```python
from build123d import *

# Parameters (mm, degrees)
SKETCH_1_R             = 2
EXTRUDE_1_DEPTH        = 5
SKETCH_2_R             = 1
CUT_EXTRUDE_1_DEPTH    = 20
PATTERN_LINEAR_1_COUNT = 14
PATTERN_LINEAR_1_PITCH = 15
FILLET_1_R             = 10
SKETCH_3_W             = 6
SKETCH_3_H             = 35
CUT_EXTRUDE_2_DEPTH    = 13
FILLET_2_R             = 3


with BuildPart() as part:
    # 草图1 → 凸台-拉伸1 (new body)
    # profile 1 of 4: a face of its own
    with BuildSketch(Plane.XY):
        with BuildLine():
            ThreePointArc((-33.2, -29.85450543), (-33.123455397, -33.472929676), (-33.700274419, -37.045902236))
            Line((-33.700274419, -37.045902236), (-46.624977248, -87.523440915))
            ThreePointArc((-46.624977248, -87.523440915), (-44.479417414, -97.858032719), (-35, -102.5))
            Line((-35, -102.5), (-5, -102.5))
            Line((-5, -102.5), (5, -102.5))
            Line((5, -102.5), (35, -102.5))
            ThreePointArc((35, -102.5), (44.479417414, -97.858032719), (46.624977248, -87.523440915))
            Line((46.624977248, -87.523440915), (33.700274419, -37.045902236))
            ThreePointArc((33.700274419, -37.045902236), (33.123455397, -33.472929676), (33.2, -29.85450543))
            Line((33.2, -29.85450543), (33.2, 7.364864087))
            Line((33.2, 7.364864087), (5, 41.001264624))
            Line((5, 41.001264624), (5, 99.5))
            ThreePointArc((5, 99.5), (4.121320344, 101.621320344), (2, 102.5))
            Line((2, 102.5), (-2.597497695, 102.5))
            ThreePointArc((-2.597497695, 102.5), (-3.665324968, 102.30352366), (-4.593283712, 101.739829943))
            Line((-4.593283712, 101.739829943), (-33.2, 76.25))
            Line((-33.2, 76.25), (-33.2, -29.85450543))
        make_face()
        with Locations((-42.25, -85.8)):
            Circle(SKETCH_1_R, mode=Mode.SUBTRACT)
        with Locations((-23.75, -85.8)):
            Circle(SKETCH_1_R, mode=Mode.SUBTRACT)
        with Locations((-9.25, -85.8)):
            Circle(SKETCH_1_R, mode=Mode.SUBTRACT)
        with Locations((-26.7, -16.25)):
            Circle(SKETCH_1_R, mode=Mode.SUBTRACT)
        with Locations((9.25, -85.8)):
            Circle(SKETCH_1_R, mode=Mode.SUBTRACT)
        with Locations((23.75, -85.8)):
            Circle(SKETCH_1_R, mode=Mode.SUBTRACT)
        with Locations((42.25, -85.8)):
            Circle(SKETCH_1_R, mode=Mode.SUBTRACT)
        with Locations((26.7, -16.25)):
            Circle(SKETCH_1_R, mode=Mode.SUBTRACT)
        with Locations((-26.7, 2.25)):
            Circle(SKETCH_1_R, mode=Mode.SUBTRACT)
        with Locations((-26.7, 53.751606034)):
            Circle(SKETCH_1_R, mode=Mode.SUBTRACT)
        with Locations((-26.45623641, 72.25)):
            Circle(SKETCH_1_R, mode=Mode.SUBTRACT)
        with Locations((26.7, 2.25)):
            Circle(SKETCH_1_R, mode=Mode.SUBTRACT)
    # profile 2 of 4: a face of its own
    with BuildSketch(Plane.XY):
        with BuildLine():
            ThreePointArc((-33.2, -29.85450543), (-33.123455397, -33.472929676), (-33.700274419, -37.045902236))
            Line((-33.700274419, -37.045902236), (-46.624977248, -87.523440915))
            ThreePointArc((-46.624977248, -87.523440915), (-44.479417414, -97.858032719), (-35, -102.5))
            Line((-35, -102.5), (-5, -102.5))
            Line((-5, -102.5), (5, -102.5))
            Line((5, -102.5), (35, -102.5))
            ThreePointArc((35, -102.5), (44.479417414, -97.858032719), (46.624977248, -87.523440915))
            Line((46.624977248, -87.523440915), (33.700274419, -37.045902236))
            ThreePointArc((33.700274419, -37.045902236), (33.123455397, -33.472929676), (33.2, -29.85450543))
            Line((33.2, -29.85450543), (33.2, 7.364864087))
            Line((33.2, 7.364864087), (5, 41.001264624))
            Line((5, 41.001264624), (5, 99.5))
            ThreePointArc((5, 99.5), (4.121320344, 101.621320344), (2, 102.5))
            Line((2, 102.5), (-2.597497695, 102.5))
            ThreePointArc((-2.597497695, 102.5), (-3.665324968, 102.30352366), (-4.593283712, 101.739829943))
            Line((-4.593283712, 101.739829943), (-33.2, 76.25))
            Line((-33.2, 76.25), (-33.2, -29.85450543))
        make_face()
        with Locations((-42.25, -85.8)):
            Circle(SKETCH_1_R, mode=Mode.SUBTRACT)
        with Locations((-23.75, -85.8)):
            Circle(SKETCH_1_R, mode=Mode.SUBTRACT)
        with Locations((-9.25, -85.8)):
            Circle(SKETCH_1_R, mode=Mode.SUBTRACT)
        with Locations((-26.7, -16.25)):
            Circle(SKETCH_1_R, mode=Mode.SUBTRACT)
        with Locations((9.25, -85.8)):
            Circle(SKETCH_1_R, mode=Mode.SUBTRACT)
        with Locations((23.75, -85.8)):
            Circle(SKETCH_1_R, mode=Mode.SUBTRACT)
        with Locations((42.25, -85.8)):
            Circle(SKETCH_1_R, mode=Mode.SUBTRACT)
        with Locations((26.7, -16.25)):
            Circle(SKETCH_1_R, mode=Mode.SUBTRACT)
        with Locations((-26.7, 2.25)):
            Circle(SKETCH_1_R, mode=Mode.SUBTRACT)
        with Locations((-26.7, 53.751606034)):
            Circle(SKETCH_1_R, mode=Mode.SUBTRACT)
        with Locations((-26.45623641, 72.25)):
            Circle(SKETCH_1_R, mode=Mode.SUBTRACT)
        with Locations((26.7, 2.25)):
            Circle(SKETCH_1_R, mode=Mode.SUBTRACT)
    # profile 3 of 4: a face of its own
    with BuildSketch(Plane.XY):
        with BuildLine():
            ThreePointArc((-33.2, -29.85450543), (-33.123455397, -33.472929676), (-33.700274419, -37.045902236))
            Line((-33.700274419, -37.045902236), (-46.624977248, -87.523440915))
            ThreePointArc((-46.624977248, -87.523440915), (-44.479417414, -97.858032719), (-35, -102.5))
            Line((-35, -102.5), (-5, -102.5))
            Line((-5, -102.5), (5, -102.5))
            Line((5, -102.5), (35, -102.5))
            ThreePointArc((35, -102.5), (44.479417414, -97.858032719), (46.624977248, -87.523440915))
            Line((46.624977248, -87.523440915), (33.700274419, -37.045902236))
            ThreePointArc((33.700274419, -37.045902236), (33.123455397, -33.472929676), (33.2, -29.85450543))
            Line((33.2, -29.85450543), (33.2, 7.364864087))
            Line((33.2, 7.364864087), (5, 41.001264624))
            Line((5, 41.001264624), (5, 99.5))
            ThreePointArc((5, 99.5), (4.121320344, 101.621320344), (2, 102.5))
            Line((2, 102.5), (-2.597497695, 102.5))
            ThreePointArc((-2.597497695, 102.5), (-3.665324968, 102.30352366), (-4.593283712, 101.739829943))
            Line((-4.593283712, 101.739829943), (-33.2, 76.25))
            Line((-33.2, 76.25), (-33.2, -29.85450543))
        make_face()
        with Locations((-42.25, -85.8)):
            Circle(SKETCH_1_R, mode=Mode.SUBTRACT)
        with Locations((-23.75, -85.8)):
            Circle(SKETCH_1_R, mode=Mode.SUBTRACT)
        with Locations((-9.25, -85.8)):
            Circle(SKETCH_1_R, mode=Mode.SUBTRACT)
        with Locations((-26.7, -16.25)):
            Circle(SKETCH_1_R, mode=Mode.SUBTRACT)
        with Locations((9.25, -85.8)):
            Circle(SKETCH_1_R, mode=Mode.SUBTRACT)
        with Locations((23.75, -85.8)):
            Circle(SKETCH_1_R, mode=Mode.SUBTRACT)
        with Locations((42.25, -85.8)):
            Circle(SKETCH_1_R, mode=Mode.SUBTRACT)
        with Locations((26.7, -16.25)):
            Circle(SKETCH_1_R, mode=Mode.SUBTRACT)
        with Locations((-26.7, 2.25)):
            Circle(SKETCH_1_R, mode=Mode.SUBTRACT)
        with Locations((-26.7, 53.751606034)):
            Circle(SKETCH_1_R, mode=Mode.SUBTRACT)
        with Locations((-26.45623641, 72.25)):
            Circle(SKETCH_1_R, mode=Mode.SUBTRACT)
        with Locations((26.7, 2.25)):
            Circle(SKETCH_1_R, mode=Mode.SUBTRACT)
    # profile 4 of 4: a face of its own
    with BuildSketch(Plane.XY):
        with BuildLine():
            ThreePointArc((-33.2, -29.85450543), (-33.123455397, -33.472929676), (-33.700274419, -37.045902236))
            Line((-33.700274419, -37.045902236), (-46.624977248, -87.523440915))
            ThreePointArc((-46.624977248, -87.523440915), (-44.479417414, -97.858032719), (-35, -102.5))
            Line((-35, -102.5), (-5, -102.5))
            Line((-5, -102.5), (5, -102.5))
            Line((5, -102.5), (35, -102.5))
            ThreePointArc((35, -102.5), (44.479417414, -97.858032719), (46.624977248, -87.523440915))
            Line((46.624977248, -87.523440915), (33.700274419, -37.045902236))
            ThreePointArc((33.700274419, -37.045902236), (33.123455397, -33.472929676), (33.2, -29.85450543))
            Line((33.2, -29.85450543), (33.2, 7.364864087))
            Line((33.2, 7.364864087), (5, 41.001264624))
            Line((5, 41.001264624), (5, 99.5))
            ThreePointArc((5, 99.5), (4.121320344, 101.621320344), (2, 102.5))
            Line((2, 102.5), (-2.597497695, 102.5))
            ThreePointArc((-2.597497695, 102.5), (-3.665324968, 102.30352366), (-4.593283712, 101.739829943))
            Line((-4.593283712, 101.739829943), (-33.2, 76.25))
            Line((-33.2, 76.25), (-33.2, -29.85450543))
        make_face()
        with Locations((-42.25, -85.8)):
            Circle(SKETCH_1_R, mode=Mode.SUBTRACT)
        with Locations((-23.75, -85.8)):
            Circle(SKETCH_1_R, mode=Mode.SUBTRACT)
        with Locations((-9.25, -85.8)):
            Circle(SKETCH_1_R, mode=Mode.SUBTRACT)
        with Locations((-26.7, -16.25)):
            Circle(SKETCH_1_R, mode=Mode.SUBTRACT)
        with Locations((9.25, -85.8)):
            Circle(SKETCH_1_R, mode=Mode.SUBTRACT)
        with Locations((23.75, -85.8)):
            Circle(SKETCH_1_R, mode=Mode.SUBTRACT)
        with Locations((42.25, -85.8)):
            Circle(SKETCH_1_R, mode=Mode.SUBTRACT)
        with Locations((26.7, -16.25)):
            Circle(SKETCH_1_R, mode=Mode.SUBTRACT)
        with Locations((-26.7, 2.25)):
            Circle(SKETCH_1_R, mode=Mode.SUBTRACT)
        with Locations((-26.7, 53.751606034)):
            Circle(SKETCH_1_R, mode=Mode.SUBTRACT)
        with Locations((-26.45623641, 72.25)):
            Circle(SKETCH_1_R, mode=Mode.SUBTRACT)
        with Locations((26.7, 2.25)):
            Circle(SKETCH_1_R, mode=Mode.SUBTRACT)
    extrude(amount=EXTRUDE_1_DEPTH)

    # 草图2 → 切除-拉伸1 (cut)
    with BuildSketch(Plane.XY):
        with Locations((0, 97.5)):
            Circle(SKETCH_2_R)
    cut_extrude_1 = extrude(amount=CUT_EXTRUDE_1_DEPTH, mode=Mode.SUBTRACT)

    # 阵列(线性)1: 切除-拉伸1 ×14
    with Locations(*[(0, -i * PATTERN_LINEAR_1_PITCH, 0) for i in range(1, PATTERN_LINEAR_1_COUNT)]):
        add(cut_extrude_1, mode=Mode.SUBTRACT)

    # 圆角1
    fillet_1_edges = [part.edges().sort_by_distance(p)[0] for p in [
        (-33.2, 76.25, 2.5),
        (5, 41.001264624, 2.5),
        (33.2, 7.364864087, 2.5),
    ]]
    fillet(fillet_1_edges, radius=FILLET_1_R)

    # 草图3 → 切除-拉伸2 (cut)
    with BuildSketch(Plane.XY):
        with Locations((-30.2, 28.069279085)):
            Rectangle(SKETCH_3_W, SKETCH_3_H)
    extrude(amount=CUT_EXTRUDE_2_DEPTH, mode=Mode.SUBTRACT)

    # 圆角2
    fillet_2_edges = [part.edges().sort_by_distance(p)[0] for p in [
        (-27.2, 45.569279085, 2.5),
        (-27.2, 10.569279085, 2.5),
    ]]
    fillet(fillet_2_edges, radius=FILLET_2_R)
    fillet_2_2_edges = [part.edges().sort_by_distance(p)[0] for p in [
        (-33.2, 45.569279085, 2.5),
        (-33.2, 10.569279085, 2.5),
    ]]
    fillet(fillet_2_2_edges, radius=FILLET_2_R - 0.0001)  # a hair under: the kernel refuses the full size


solid = part.part
```
Work out the finished part from the listing and answer in its coordinate system (mm). A direction names the side the tool comes from. Round coordinates to 2 decimals unless told otherwise and drop trailing zeros. Loops run counter-clockwise (first coordinate to the right, second up) from the corner with the lowest first, then second, coordinate; pieces in that order, holes last. Notation, with made-up numbers: (54.25, 78) -> (94.25, 78) arc R12 cw to (94.25, 87) -> close; hole circle Ø10 at (-26.75, 38). An arc over 180 degrees is marked (long way). Write each question's results on one line, items separated by ' | '. Start each with the question number.
1. Given pin 1 Ø2 at (y, z) = (-60.5, 1) entering from -X; pin 2 Ø2.5 at (y, z) = (31, 1.5) entering from -X; pin 3 Ø2.5 at (y, z) = (-19.5, 1.5) entering from +X, each flat-ended and moving along its own axis, determine where each tip first touches the part or whether it passes through.
2. Section B-B (x = 9.25) is taken. Determine the outline of the cut face in (y, z), plus the area to 3 significant figures.
3. Section D-D (y = 18) is taken. Determine the outline of the cut face in (x, z), plus the area to 3 significant figures.
4. A tool of negligible diameter and unlimited length cuts with its end or side. For faces 4 (the face through (-27.2, 28, 2)), 5 (the face through (-33.2, 60, 2)), 6 (the face through (33.127, -33.524, 2.465)), from which of +Z, -Z, +X, -X, +Y, -Y can it reach the whole face along a straight path? Write none if from no direction.
5. Find the intervals of material crossed by probe 1 along Y at (x, z) = (26.7, 2.8); probe 2 along X at (y, z) = (1, 0.5); probe 3 along X at (y, z) = (-31.5, 2.05), in increasing order. Write a range as from..to.
6. Section C-C (z = 1.25) is taken. State how many separate pieces and enclosed holes the cut face has, plus the area to 3 significant figures.
7. For a pull along Y with two mould halves and no side action, classify faces 1 (the face through (5, 72, 2)), 2 (the face through (28.547, 1.484, 2.465)), 3 (the face through (32.58, 7.19, 2.54)) as +Y half, -Y half, draft (parallel to the pull), parting line (faces both ways), or undercut.
8. Section A-A (y = -16.25) is taken. Determine the outline of the cut face in (x, z).
Evaluation:
1) pin 1: stops at x = -39.96 | pin 2: stops at x = -27.2 | pin 3: stops at x = 33.2
2) outline: (-102.5, 0) -> (-87.8, 0) -> (-87.8, 5) -> (-102.5, 5) -> close; (-83.8, 0) -> (35.93, 0) -> (35.93, 5) -> (-83.8, 5) -> close | area: 672 mm2
3) outline: (-27.2, 0) -> (24.28, 0) -> (24.28, 5) -> (-27.2, 5) -> close | area: 257 mm2
4) face 4: +Z, -Z, -X | face 5: +Z, -Z, -X, +Y | face 6: +Z, -Z, +X
5) probe 1: y = -102.5..-18.25, -14.25..0.25, 4.25..15.12 | probe 2: x = -33.2..-28.26, -25.14..25.14, 28.26..33.2 | probe 3: x = -33.08..33.08
6) separate pieces: 1 | enclosed holes: 26 | area: 11,700 mm2
7) face 1: draft | face 2: undercut | face 3: +Y half
8) outline: (-33.2, 0) -> (-28.7, 0) -> (-28.7, 5) -> (-33.2, 5) -> close; (-24.7, 0) -> (24.7, 0) -> (24.7, 5) -> (-24.7, 5) -> close; (28.7, 0) -> (33.2, 0) -> (33.2, 5) -> (28.7, 5) -> close
